Verification items for this drawing (mm, ordinates from the low corner). A direction names the side the tool comes from. Give positions to 0.01 mm unless a question says otherwise; leave off trailing zeros. Order: outer loops, then holes, each group sorted by start corner. A loop starts at its lowest first (then second) coordinate and runs counter-clockwise, first axis right, second up. Notation, with made-up numbers: M 86,74 L 127,74 A24 cw 127,111 Z; hole C -27,-15.5 d6. An arc over 180 degrees is marked long. Answer as a JSON object with one key per item and string values.
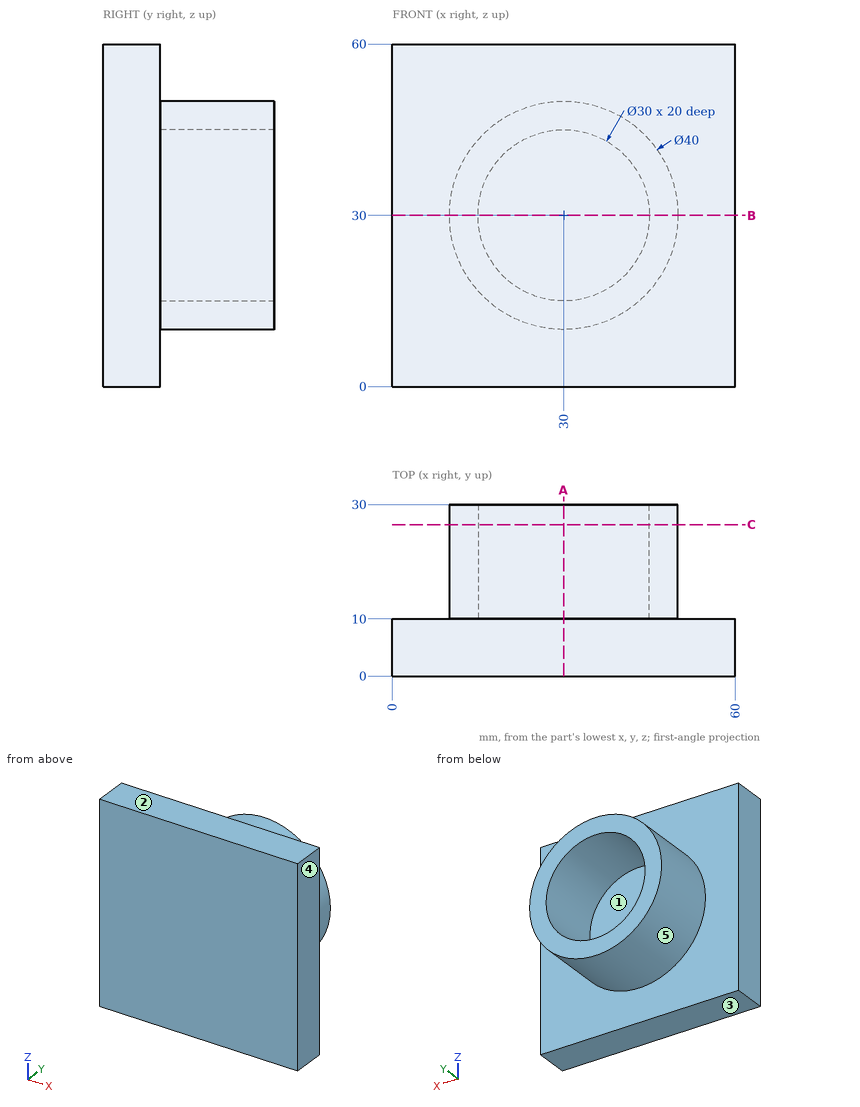
Q1. Gauge pin test, flat ends, axial feed: pin 1 Ø24 at (x, z) = (28, 28) entering from +Y; pin 2 Ø3 at (x, y) = (13.5, 26) entering from +Z; pin 3 Ø5 at (y, z) = (26.5, 38) entering from -X; pin 4 Ø3 at (x, z) = (49.5, 10) entering from -Y. Record the tip position at first contact, or that the pin passes through.
Resolved:
{"pin 1": "stops at y = 10", "pin 2": "stops at z = 43.23", "pin 3": "stops at x = 10.77", "pin 4": "stops at y = 0"}
Q2. Section check C-C on y = 26.5. Record the cut outline in (x, z).
Resolved:
{"outline": "C 30,30 d40; hole C 30,30 d30"}
Q3. Section check A-A on x = 30. Record the cut outline in (y, z), then the cut area to 3 significant figures.
Resolved:
{"outline": "M 0,0 L 10,0 L 10,10 L 30,10 L 30,15 L 10,15 L 10,45 L 30,45 L 30,50 L 10,50 L 10,60 L 0,60 Z", "area": "800 mm²"}
Q4. Release check for a two-part mould opening along Z. For the marked faces 1, 2 and 3 record: +Z half, -Z half, draft (parallel to the pull), parting line (faces both ways), or undercut.
Resolved:
{"face 1": "undercut", "face 2": "+Z half", "face 3": "-Z half"}
Q5. Section check B-B on z = 30. Record the cut outline in (x, y), then the cut area to 3 significant figures.
Resolved:
{"outline": "M 0,0 L 60,0 L 60,10 L 50,10 L 50,30 L 45,30 L 45,10 L 15,10 L 15,30 L 10,30 L 10,10 L 0,10 Z", "area": "800 mm²"}
Q6. Tool access check on the marked faces 4 and 5. Record the directions out of +Z, -Z, +X, -X, +Y, -Y that give a thin tool (end or side, any length) a straight path to the whole face; none if there is none.
Resolved:
{"face 4": "+Z, -Z, +X, +Y, -Y", "face 5": "+Y"}
Q7. Material ranges on L1, parallel to X at y = 18.25, z = 30; L2, parallel to Y at x = 29, z = 32, recorded low to high.
Resolved:
{"L1": "x = 10 to 15, 45 to 50", "L2": "y = 0 to 10"}
